```python
from build123d import *

# Parameters (mm, degrees)
SKETCH1_R           = 300
SKETCH1_R_2         = 270
BOSS_EXTRUDE1_DEPTH = 50
FILLET1_R           = 25
SHELL1_T            = -2


with BuildPart() as part:
    # Sketch1 → Boss-Extrude1 (new body)
    with BuildSketch(Plane(origin=(0, 0, 0), x_dir=(0, 0, -1), z_dir=(1, 0, 0))):
        Circle(SKETCH1_R)
        Circle(SKETCH1_R_2, mode=Mode.SUBTRACT)
    extrude(amount=BOSS_EXTRUDE1_DEPTH)

    # Fillet1
    fillet1_edges = [part.edges().sort_by_distance(p)[0] for p in [
        (0, 0, 300),
        (50, 0, 300),
    ]]
    fillet(fillet1_edges, radius=FILLET1_R - 0.0001)  # a hair under: the kernel refuses the full size

    # Shell1
    shell1_openings = [part.faces().sort_by_distance(p)[0] for p in [
        (25, 0, 270),
    ]]
    offset(amount=SHELL1_T, openings=shell1_openings, kind=Kind.INTERSECTION)


solid = part.part
```
The listing builds one solid part. Answer for the finished solid, in the listing's coordinates (mm). A direction names the side the tool comes from. Round coordinates to 2 decimals unless told otherwise and drop trailing zeros. Loops run counter-clockwise (first coordinate to the right, second up) from the corner with the lowest first, then second, coordinate; pieces in that order, holes last.
Q1. Find the intervals of material crossed by line 1 (Y direction, x = 25, z = 0); line 2 (Y direction, x = 40, z = -46.5); line 3 (Z direction, x = 42.5, y = -142.5), in increasing order.
Q2. For a pull along X with two mould halves and no side action, classify faces 3 (the face through (2, -202, -182)), 4 (the face through (50, -202, -182)), 5 (the face through (0.986, -164.291, 214.263)) as released by +X, released by -X, zero draft, split by the parting line, or undercut.
Q3. Section C-C, the plane x = 33 is taken. Determine the outline of the cut face in (y, z).
Q4. Given pin 1 Ø1.5 at (x, y) = (17, 106) entering from +Z; pin 2 Ø1.5 at (x, z) = (39.5, -184.5) entering from -Y; pin 3 Ø2 at (x, y) = (16, -235.5) entering from -Z, each flat-ended and moving along its own axis, determine where each tip first touches the part or whether it passes through.
Q5. Which of the six approach directions +Z, -Z, +X, -X, +Y, -Y give full straight-line access (tool end or side, diameter ignored) to faces 1 (the face through (48, -202, -182)), 2 (the face through (0, -202, -182))?
Completed:
1. line 1: y = -300 to -298, 298 to 300
1. line 2: y = -291.31 to -288.72, 288.72 to 291.31
1. line 3: z = -255.85 to -252.49, 252.49 to 255.85
2. face 3: undercut
2. face 4: released by +X
2. face 5: zero draft
3. outline: circle Ø597.37 at (0, 0); hole circle Ø593.13 at (0, 0)
4. pin 1: stops at z = 279.63
4. pin 2: stops at y = -231.55
4. pin 3: stops at z = -184.55
5. face 1: none
5. face 2: +Z, -Z, -X, +Y, -Y
